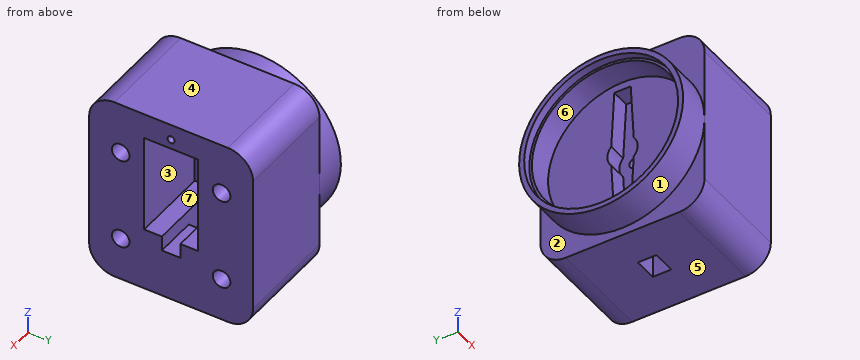
```python
from build123d import *

# Parameters (mm, degrees)
SKETCH1_W           = 40.7
SKETCH1_H           = 17
BOSS_EXTRUDE1_DEPTH = 24.5
SKETCH2_W           = 40.7
SKETCH2_H           = 34
BOSS_EXTRUDE2_DEPTH = 4
SKETCH3_R           = 3.6
CUT_EXTRUDE1_DEPTH  = 4.4
CUT_EXTRUDE2_DEPTH  = 4.4
SKETCH5_R           = 1.2
CUT_EXTRUDE3_DEPTH  = 7
SKETCH6_W           = 23.4
SKETCH6_H           = 12.8
CUT_EXTRUDE4_DEPTH  = 19.2
SKETCH7_W           = 3.7
SKETCH7_H           = 4.4
CUT_EXTRUDE5_DEPTH  = 16
SKETCH8_R           = 0.85
CUT_EXTRUDE6_DEPTH  = 8.6
SKETCH9_R           = 1.7
CUT_EXTRUDE7_DEPTH  = 4.7
SKETCH10_W          = 5.5
SKETCH10_H          = 4.4
CUT_EXTRUDE8_DEPTH  = 8.3
BOSS_EXTRUDE3_DEPTH = 24.5
SKETCH12_W          = 5.5
SKETCH12_H          = 4.4
CUT_EXTRUDE9_DEPTH  = 3.5
CUT_EXTRUDE10_DEPTH = 326.708673511
SKETCH14_R          = 19.5
SKETCH14_R_2        = 18.3
BOSS_EXTRUDE4_DEPTH = 7.9
SKETCH15_R          = 2.1
CUT_EXTRUDE11_DEPTH = 6.1
SKETCH16_R          = 18.3
SKETCH16_R_2        = 17.7
BOSS_EXTRUDE6_DEPTH = 6


with BuildPart() as part:
    # Sketch1 → Boss-Extrude1 (new body)
    with BuildSketch(Plane(origin=(169.4, 0, 0), x_dir=(0, 0, -1), z_dir=(1, 0, 0))):
        with Locations((-303.85, 0)):
            Rectangle(SKETCH1_W, SKETCH1_H)
    extrude(amount=BOSS_EXTRUDE1_DEPTH)

    # Sketch2 → Boss-Extrude2 (add)
    with BuildSketch(Plane(origin=(189.9, 0, 0), x_dir=(0, 0, -1), z_dir=(1, 0, 0))):
        with Locations((-303.85, 0)):
            Rectangle(SKETCH2_W, SKETCH2_H)
    extrude(amount=BOSS_EXTRUDE2_DEPTH)

    # Sketch3 → Cut-Extrude1 (cut)
    with BuildSketch(Plane(origin=(169.4, 0, 0), x_dir=(0, 0, -1), z_dir=(1, 0, 0))):
        with Locations((-301, 0)):
            Circle(SKETCH3_R)
    extrude(amount=CUT_EXTRUDE1_DEPTH, mode=Mode.SUBTRACT)

    # Sketch4 → Cut-Extrude2 (cut)
    with BuildSketch(Plane(origin=(169.4, 0, 0), x_dir=(0, 0, -1), z_dir=(1, 0, 0))):
        Polygon((-285.15, -1.95), (-301, -2.8), (-316.85, -1.95), (-316.85, 1.95), (-301, 2.8), (-285.15, 1.95), align=None)
    extrude(amount=CUT_EXTRUDE2_DEPTH, mode=Mode.SUBTRACT)

    # Sketch5 → Cut-Extrude3 (cut)
    with BuildSketch(Plane(origin=(169.4, 0, 0), x_dir=(0, 0, -1), z_dir=(1, 0, 0))):
        with Locations((-301, 0)):
            Circle(SKETCH5_R)
    extrude(amount=CUT_EXTRUDE3_DEPTH, mode=Mode.SUBTRACT)

    # Sketch6 → Cut-Extrude4 (cut)
    with BuildSketch(Plane(origin=(194.5, 0, 0), x_dir=(0, 0, -1), z_dir=(1, 0, 0))):
        with Locations((-306.45, 0)):
            Rectangle(SKETCH6_W, SKETCH6_H)
    extrude(amount=-CUT_EXTRUDE4_DEPTH, mode=Mode.SUBTRACT)

    # Sketch7 → Cut-Extrude5 (cut)
    with BuildSketch(Plane(origin=(194.5, 0, 0), x_dir=(0, 0, -1), z_dir=(1, 0, 0))):
        with Locations((-293.05, 0)):
            Rectangle(SKETCH7_W, SKETCH7_H)
    extrude(amount=-CUT_EXTRUDE5_DEPTH, mode=Mode.SUBTRACT)

    # Sketch8 → Cut-Extrude6 (cut)
    with BuildSketch(Plane(origin=(194.5, 0, 0), x_dir=(0, 0, -1), z_dir=(1, 0, 0))):
        with Locations((-320.45, 0)):
            Circle(SKETCH8_R)
    extrude(amount=-CUT_EXTRUDE6_DEPTH, mode=Mode.SUBTRACT)

    # Sketch9 → Cut-Extrude7 (cut)
    with BuildSketch(Plane(origin=(194.5, 0, 0), x_dir=(0, 0, -1), z_dir=(1, 0, 0))):
        with Locations(Location((-290, 12, 0), (0, 0, 180))):
            Circle(SKETCH9_R)
        with Locations(Location((-290, -12, 0), (0, 0, 180))):
            Circle(SKETCH9_R)
        with Locations(Location((-312, 12, 0), (0, 0, 180))):
            Circle(SKETCH9_R)
        with Locations(Location((-312, -12, 0), (0, 0, 180))):
            Circle(SKETCH9_R)
    extrude(amount=-CUT_EXTRUDE7_DEPTH, mode=Mode.SUBTRACT)

    # Sketch10 → Cut-Extrude8 (cut)
    with BuildSketch(Plane.XY.offset(283)):
        with Locations((181.25, 0)):
            Rectangle(SKETCH10_W, SKETCH10_H)
    extrude(amount=CUT_EXTRUDE8_DEPTH, mode=Mode.SUBTRACT)

    # Sketch11 → Boss-Extrude3 (add)
    with BuildSketch(Plane(origin=(169.4, 0, 0), x_dir=(0, 0, -1), z_dir=(1, 0, 0))):
        Polygon((-279.7, -19.5), (-324.2, -19.5), (-324.2, -8.5), (-283.5, -8.5), (-283.5, 8.5), (-324.2, 8.5), (-324.2, 19.5), (-279.7, 19.5), align=None)
    extrude(amount=BOSS_EXTRUDE3_DEPTH)

    # Sketch12 → Cut-Extrude9 (cut, symmetric)
    with BuildSketch(Plane.XY.offset(283)):
        with Locations((181.25, 0)):
            Rectangle(SKETCH12_W, SKETCH12_H)
    extrude(amount=CUT_EXTRUDE9_DEPTH, both=True, mode=Mode.SUBTRACT)

    # Sketch13 → Cut-Extrude10 (cut, through all)
    with BuildSketch(Plane(origin=(169.4, 0, 0), x_dir=(0, 0, -1), z_dir=(1, 0, 0))):
        with BuildLine():
            Line((-324.2, 13.5), (-325.5, 13.5))
            Line((-325.5, 13.5), (-325.5, 20.5))
            Line((-325.5, 20.5), (-318.2, 20.5))
            Line((-318.2, 20.5), (-318.2, 19.5))
            ThreePointArc((-318.2, 19.5), (-322.442640687, 17.742640687), (-324.2, 13.5))
        make_face()
        with BuildLine():
            Line((-324.2, -13.5), (-325.5, -13.5))
            Line((-325.5, -13.5), (-325.5, -20.5))
            Line((-325.5, -20.5), (-318.2, -20.5))
            Line((-318.2, -20.5), (-318.2, -19.5))
            ThreePointArc((-318.2, -19.5), (-322.442640687, -17.742640687), (-324.2, -13.5))
        make_face()
        with BuildLine():
            Line((-279.7, 13.5), (-278.4, 13.5))
            Line((-278.4, 13.5), (-278.4, 20.5))
            Line((-278.4, 20.5), (-285.7, 20.5))
            Line((-285.7, 20.5), (-285.7, 19.5))
            ThreePointArc((-285.7, 19.5), (-281.457359313, 17.742640687), (-279.7, 13.5))
        make_face()
        with BuildLine():
            Line((-279.7, -13.5), (-278.4, -13.5))
            Line((-278.4, -13.5), (-278.4, -20.5))
            Line((-278.4, -20.5), (-285.7, -20.5))
            Line((-285.7, -20.5), (-285.7, -19.5))
            ThreePointArc((-285.7, -19.5), (-281.457359313, -17.742640687), (-279.7, -13.5))
        make_face()
    extrude(amount=CUT_EXTRUDE10_DEPTH, mode=Mode.SUBTRACT)

    # Sketch14 → Boss-Extrude4 (add)
    with BuildSketch(Plane(origin=(169.4, 0, 0), x_dir=(0, 0, -1), z_dir=(1, 0, 0))):
        with Locations((-301, 0)):
            Circle(SKETCH14_R)
        with Locations((-301, 0)):
            Circle(SKETCH14_R_2, mode=Mode.SUBTRACT)
    extrude(amount=-BOSS_EXTRUDE4_DEPTH)

    # Sketch15 → Cut-Extrude11 (cut)
    with BuildSketch(Plane(origin=(194.5, 0, 0), x_dir=(0, 0, -1), z_dir=(1, 0, 0))):
        with Locations((-290, 12)):
            Circle(SKETCH15_R)
        with Locations((-290, -12)):
            Circle(SKETCH15_R)
        with Locations((-312, 12)):
            Circle(SKETCH15_R)
        with Locations((-312, -12)):
            Circle(SKETCH15_R)
    extrude(amount=-CUT_EXTRUDE11_DEPTH, mode=Mode.SUBTRACT)

    # Sketch16 → Boss-Extrude6 (add)
    with BuildSketch(Plane(origin=(169.4, 0, 0), x_dir=(0, 0, -1), z_dir=(1, 0, 0))):
        with Locations((-301, 0)):
            Circle(SKETCH16_R)
        with Locations((-301, 0)):
            Circle(SKETCH16_R_2, mode=Mode.SUBTRACT)
    extrude(amount=-BOSS_EXTRUDE6_DEPTH)


solid = part.part
```
Geometry check sheet. Reference: the model listing, model coordinates, mm. Face numbers are marked on the shaded views. A direction names the side the tool comes from. Coordinates: 2 decimals unless noted, no trailing zeros. Order: outer loops, then holes, each group sorted by start corner. A loop starts at its lowest first (then second) coordinate and runs counter-clockwise, first axis right, second up. Notation, with made-up numbers: (25, 82.25) - (70, 82.25) arc R32 ccw to (70, 111.25) - close; hole circle Ø11 at (-36, -10.5). An arc over 180 degrees is marked (long way). Answer in a Markdown table with one row per item. Add a question column.
1. Access from +Z, -Z, +X, -X, +Y, -Y to the whole of each face (thin tool, end or side, straight path). Record for the marked faces 1, 2 and 3.
2. Material ranges on L1, parallel to Y at x = 192, z = 290; L2, parallel to Y at x = 191.2, z = 312; L3, parallel to Z at x = 190.5, y = -5.5, recorded low to high. Write a range as [from, to].
3. Section check A-A (y = 0). Give the number of separate pieces and of enclosed holes in the cut face, plus the area to 3 significant figures.
4. Gauge pin test, flat ends, axial feed: pin 1 Ø12 at (x, z) = (165, 317.5) entering from +Y; pin 2 Ø2 at (y, z) = (11.5, 290) entering from +X; pin 3 Ø0.5 at (y, z) = (-0.5, 320.5) entering from +X; pin 4 Ø1.3 at (y, z) = (-1, 286.5) entering from -X. Record the tip position at first contact, or that the pin passes through.
5. Section check B-B (x = 183). Enter the section's corners in (y, z), plus the area to 3 significant figures.
6. Draft check along Z on the marked faces 4, 5, 6 and 7. Enter one of: +Z half, -Z half, draft (parallel to the pull), parting line (faces both ways), or undercut.
7. Section check D-D (y = 7.5). Enter the section's corners in (x, z).
Data:
| question | item | result |
|---|---|---|
| 1 | face 1 | -X |
| 1 | face 2 | -Z, -X |
| 1 | face 3 | +X |
| 2 | L1 | y = [-19.5, -14.1], [-9.9, 9.9], [14.1, 19.5] |
| 2 | L2 | y = [-19.5, -14.1], [-9.9, -6.4], [6.4, 9.9], [14.1, 19.5] |
| 2 | L3 | z = [279.7, 294.75], [318.15, 324.2] |
| 3 | separate pieces | 3 |
| 3 | enclosed holes | 0 |
| 3 | area | 407 mm² |
| 4 | pin 1 | stops at y = 19.5 |
| 4 | pin 2 | stops at x = 188.4 |
| 4 | pin 3 | stops at x = 185.9 |
| 4 | pin 4 | stops at x = 173.8 |
| 5 | outline | (-19.5, 285.7) arc R6 ccw to (-13.5, 279.7) - (-2.2, 279.7) - (-2.2, 294.75) - (-6.4, 294.75) - (-6.4, 318.15) - (6.4, 318.15) - (6.4, 294.75) - (2.2, 294.75) - (2.2, 279.7) - (13.5, 279.7) arc R6 ccw to (19.5, 285.7) - (19.5, 318.2) arc R6 ccw to (13.5, 324.2) - (-13.5, 324.2) arc R6 ccw to (-19.5, 318.2) - close |
| 5 | area | 1,340 mm² |
| 6 | face 4 | +Z half |
| 6 | face 5 | -Z half |
| 6 | face 6 | undercut |
| 6 | face 7 | undercut |
| 7 | outline | (161.5, 283) - (169.4, 283) - (169.4, 279.7) - (193.9, 279.7) - (193.9, 324.2) - (169.4, 324.2) - (169.4, 319) - (161.5, 319) - (161.5, 317.69) - (163.4, 317.69) - (163.4, 317.03) - (169.4, 317.03) - (169.4, 284.97) - (163.4, 284.97) - (163.4, 284.31) - (161.5, 284.31) - close |
